Model file for the job. Use its own axes, mm. A direction names the side the tool comes from. Round coordinates to 2 decimals unless told otherwise and drop trailing zeros. Order: outer loops, then holes, each group sorted by start corner. A loop starts at its lowest first (then second) coordinate and runs counter-clockwise, first axis right, second up. Notation, with made-up numbers: (54, 27) - (91, 27) arc R10 cw to (91, 43) - close; hole circle Ø11 at (17.25, 53.25). An arc over 180 degrees is marked (long way). Write item = value, one per line.
```python
from build123d import *

# Parameters (mm, degrees)
SKETCH4_W           = 50
SKETCH4_H           = 50
BOSS_EXTRUDE1_DEPTH = 10
SKETCH5_W           = 40
SKETCH5_H           = 40
CUT_EXTRUDE1_DEPTH  = 7
SKETCH9_W           = 5
SKETCH9_H           = 5
SKETCH9_R           = 1.5
BOSS_EXTRUDE4_DEPTH = 1


with BuildPart() as part:
    # Sketch4 → Boss-Extrude1 (new body)
    with BuildSketch(Plane(origin=(0, 0, 0), x_dir=(1, 0, 0), z_dir=(0, 1, 0))):
        Rectangle(SKETCH4_W, SKETCH4_H)
    extrude(amount=BOSS_EXTRUDE1_DEPTH)

    # Sketch5 → Cut-Extrude1 (cut)
    with BuildSketch(Plane(origin=(0, 0, 0), x_dir=(1, 0, 0), z_dir=(0, 1, 0))):
        Rectangle(SKETCH5_W, SKETCH5_H)
    extrude(amount=CUT_EXTRUDE1_DEPTH, mode=Mode.SUBTRACT)

    # Sketch9 → Boss-Extrude4 (add)
    with BuildSketch(Plane.XZ):
        with Locations((-22.5, -27.5)):
            Rectangle(SKETCH9_W, SKETCH9_H)
        with Locations(Location((-22.5, -27.5, 0), (0, 0, 270))):  # turned: the seam where the file's is
            Circle(SKETCH9_R, mode=Mode.SUBTRACT)
        with Locations((22.5, 27.5)):
            Rectangle(SKETCH9_W, SKETCH9_H)
        with Locations(Location((22.5, 27.5, 0), (0, 0, 270))):  # turned: the seam where the file's is
            Circle(SKETCH9_R, mode=Mode.SUBTRACT)
    extrude(amount=-BOSS_EXTRUDE4_DEPTH)


solid = part.part
```
1) Wall check: line 1 along X through (y, z) = (0.4, 27.5); line 2 along X through (y, z) = (0.35, -27.5); line 3 along Z through (x, y) = (-15.5, 6.75). Give the ranges that are in metal, low to high.
Conclusion:
line_1 = 20 to 21, 24 to 25
line_2 = -25 to -24, -21 to -20
line_3 = -25 to -20, 20 to 25
2) Cut at A-A (z = 27.5). Write the cut outline in (x, y), and give its area (3 significant figures).
Conclusion:
outline = (20, 0) - (21, 0) - (21, 1) - (20, 1) - close; (24, 0) - (25, 0) - (25, 1) - (24, 1) - close
area = 2.00 mm^2
3) Cut at D-D (x = 3.5). Write the cut outline in (y, z), and give its area (3 significant figures).
Conclusion:
outline = (0, -25) - (10, -25) - (10, 25) - (0, 25) - (0, 20) - (7, 20) - (7, -20) - (0, -20) - close
area = 220 mm^2
4) Cut at B-B (x = -22.5). Write the cut outline in (y, z), and give its area (3 significant figures).
Conclusion:
outline = (0, -30) - (1, -30) - (1, -29) - (0, -29) - close; (0, -26) - (1, -26) - (1, -25) - (10, -25) - (10, 25) - (0, 25) - close
area = 502 mm^2
5) Mould opens along X. For faces 5 (the face through (23.51, 0.49, 28.61)), 6 (the face through (-20, 3, 0)), 7 (the face through (-20.5, 0, 2.4)), 8 (the face through (-25, 5, -3)) say: +X half, -X half, draft (parallel to the pull), parting line (faces both ways), or undercut.
Conclusion:
face_5 = undercut
face_6 = undercut
face_7 = draft
face_8 = -X half
6) Flat gauge pins, fed straight in: pin 1 Ø20 at (x, z) = (-8, 1.5) entering from -Y; pin 2 Ø1.5 at (x, y) = (19, 8.5) entering from -Z; pin 3 Ø4 at (x, z) = (-23, -28) entering from +Y. Where does each tip first touch, or does it go through?
Conclusion:
pin_1 = 7
pin_2 = -25
pin_3 = 1
7) Cut at C-C (y = 5). Write the cut outline in (x, z), and give its area (3 significant figures).
Conclusion:
outline = (-25, -25) - (25, -25) - (25, 25) - (-25, 25) - close; hole (-20, -20) - (20, -20) - (20, 20) - (-20, 20) - close
area = 900 mm^2
8) 3-axis set-ups, long thin cutter, end or side, ignore diameter. For faces 1 (the face through (20, 3, 0)), 2 (the face through (-21, 1, -26)), 3 (the face through (0, 10, 0)), 4 (the face through (24, 1, 29)): which of +Z, -Z, +X, -X, +Y, -Y reach the whole face in a straight line?
Conclusion:
face_1 = -Y
face_2 = -Z, +X, -X, +Y
face_3 = +Z, -Z, +X, -X, +Y
face_4 = +Z, +X, -X, +Y
